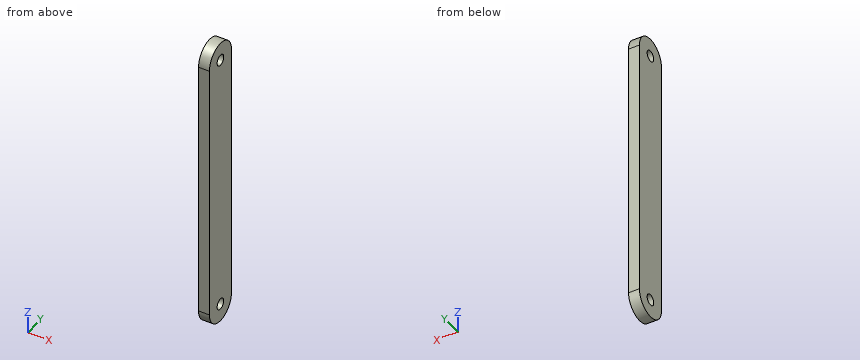
```python
from build123d import *

# Parameters (mm, degrees)
BOSS_EXTRUDE1_DEPTH      = 36.25
BOSS_EXTRUDE1_DEPTH_BACK = 36.25
SKETCH2_W                = 3
SKETCH2_H                = 10
SKETCH3_W                = 3
SKETCH3_H                = 5
SKETCH4_R                = 1.5
CUT_EXTRUDE1_DEPTH       = 3


with BuildPart() as part:
    # Sketch2 → Boss-Extrude1 (new, two sides: drawn at the far end of the back side and taken through both)
    with BuildSketch(Plane.XY.offset(-BOSS_EXTRUDE1_DEPTH_BACK)):
        Rectangle(SKETCH2_W, SKETCH2_H)
    extrude(amount=BOSS_EXTRUDE1_DEPTH + BOSS_EXTRUDE1_DEPTH_BACK)

    # Sketch3 → Revolve1 (revolve)
    with BuildSketch(Plane(origin=(0, 0, -36.25), x_dir=(-1, 0, 0), z_dir=(0, 0, -1))):
        with Locations((0, -2.5)):
            Rectangle(SKETCH3_W, SKETCH3_H)
    revolve1 = revolve(axis=Axis((-1.5, 0, -36.25), (1, 0, 0)))

    # Sketch4 → Cut-Extrude1 (cut)
    with BuildSketch(Plane(origin=(1.5, 0, 0), x_dir=(0, 0, -1), z_dir=(1, 0, 0))):
        with Locations(Location((36.25, 0, 0), (0, 0, 90))):
            Circle(SKETCH4_R)
    cut_extrude1 = extrude(amount=-CUT_EXTRUDE1_DEPTH, mode=Mode.SUBTRACT)

    # Mirror1: Revolve1, Cut-Extrude1 across plane
    add(revolve1.mirror(Plane.XY))
    add(cut_extrude1.mirror(Plane.XY), mode=Mode.SUBTRACT)


solid = part.part
```
Geometry check sheet. Reference: the model listing, model coordinates, mm. Give positions to 0.01 mm unless a question says otherwise; leave off trailing zeros. Order: outer loops, then holes, each group sorted by start corner. A loop starts at its lowest first (then second) coordinate and runs counter-clockwise, first axis right, second up. Notation, with made-up numbers: (4.25, 85) -> (56.25, 85) arc R21 cw to (56.25, 111) -> close; hole circle Ø2 at (84.25, -6.5). An arc over 180 degrees is marked (long way). Write each question's results on one line, items separated by ' | '. Start each with the question number.
(1) Scan lines: line 1 (Z direction, x = -0.2, y = 0); line 2 (Y direction, x = 0.65, z = 36.25); line 3 (Z direction, x = -0.25, y = 3.75). Record each from-to range of solid material in increasing order.
(2) Sectioned sample at A-A (x = -0.8). Enter the section's corners in (y, z).
(3) Sectioned sample at C-C (y = 4). Enter the section's corners in (x, z).
(4) Sectioned sample at B-B (y = 0). Enter the section's corners in (x, z), plus the area to 4 significant figures.
(5) Gauge pin test, flat ends, axial feed: P1, Ø5, axis at y = 0, z = 36.25, coming from the -X side; P2, Ø1, axis at x = 1, y = 3.5, coming from the -Z side; P3, Ø1.5, axis at x = -0.5, y = -3.5, coming from the -Z side. Record the tip position at first contact, or that the pin passes through.
Answer below:
1) line 1: -41.25 to -37.75, -34.75 to 34.75, 37.75 to 41.25 | line 2: -5 to -1.5, 1.5 to 5 | line 3: -39.56 to 39.56
2) outline: (-5, -36.25) arc R5 ccw to (5, -36.25) -> (5, 36.25) arc R5 ccw to (-5, 36.25) -> close; hole circle Ø3 at (0, -36.25); hole circle Ø3 at (0, 36.25)
3) outline: (-1.5, -39.25) -> (1.5, -39.25) -> (1.5, 39.25) -> (-1.5, 39.25) -> close
4) outline: (-1.5, -41.25) -> (1.5, -41.25) -> (1.5, -37.75) -> (-1.5, -37.75) -> close; (-1.5, -34.75) -> (1.5, -34.75) -> (1.5, 34.75) -> (-1.5, 34.75) -> close; (-1.5, 37.75) -> (1.5, 37.75) -> (1.5, 41.25) -> (-1.5, 41.25) -> close | area: 229.5 mm2
5) P1: x = -1.5 | P2: z = -40.25 | P3: z = -40.43
